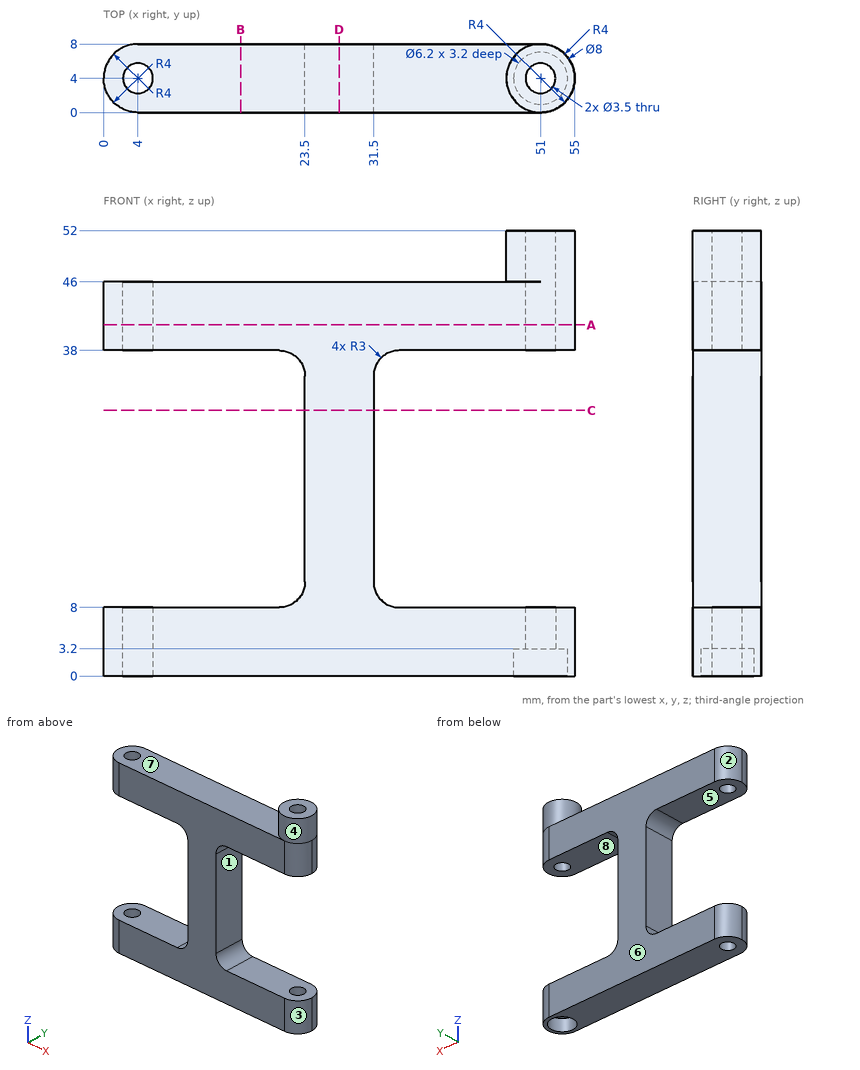
Geometry check sheet. Reference: drawing and pictorial views, mm from the part's lowest x, y, z. A direction names the side the tool comes from. Round coordinates to 2 decimals unless told otherwise and drop trailing zeros. Loops run counter-clockwise (first coordinate to the right, second up) from the corner with the lowest first, then second, coordinate; pieces in that order, holes last. Notation, with made-up numbers: (89.25, 13.25) - (93.25, 13.25) arc R27 ccw to (93.25, 48.25) - close; hole circle Ø4 at (19, 85). An arc over 180 degrees is marked (long way). Write item = value, one per line. Start each with the question number.
Q1. Section check C-C (z = 31). Record the boundary of the cut face in (x, y).
Q2. Section check A-A (z = 41). Count the separate pieces of the cut face and the enclosed holes in it, plus the area to 3 significant figures.
Q3. Section check B-B (x = 16). Record the boundary of the cut face in (y, z), plus the area to 3 significant figures.
Q4. Access from +Z, -Z, +X, -X, +Y, -Y to the whole of each face (thin tool, end or side, straight path). Record for the marked faces 1, 2, 3, 4 and 5.
Q5. Section check D-D (x = 27.5). Record the boundary of the cut face in (y, z), plus the area to 3 significant figures.
Q6. Depth check by flat-ended pin: P1, Ø4, axis at x = 4, y = 4, coming from the +Z side; P2, Ø4, axis at y = 6, z = 27.5, coming from the -X side. Enter the tip coordinate at first touch or a pass-through.
Q7. Thickness scan on L1, parallel to Z at x = 16.5, y = 3.75; L2, parallel to Y at x = 4, z = 5; L3, parallel to X at y = 3.75, z = 42. Record the ranges inside material, lowest first.
Q8. Release check for a two-part mould opening along Z. For the marked faces 6, 7 and 8 record: pulls with the +Z half, pulls with the -Z half, needs draft (parallel to the pull), parting line crosses it, or undercut.
Derived:
q1.outline = (23.5, 0) - (31.5, 0) - (31.5, 8) - (23.5, 8) - close
q2.separate_pieces = 1
q2.enclosed_holes = 2
q2.area = 407 mm^2
q3.outline = (0, 0) - (8, 0) - (8, 8) - (0, 8) - close; (0, 38) - (8, 38) - (8, 46) - (0, 46) - close
q3.area = 128 mm^2
q4.face_1 = +X, +Y, -Y
q4.face_2 = +Z, -Z, -X, +Y
q4.face_3 = +Z, -Z, +X, -Y
q4.face_4 = +Z
q4.face_5 = -X, +Y, -Y
q5.outline = (0, 0) - (8, 0) - (8, 46) - (0, 46) - close
q5.area = 368 mm^2
q6.P1 = 46
q6.P2 = 23.5
q7.L1 = 0 to 8, 38 to 46
q7.L2 = 0 to 2.25, 5.75 to 8
q7.L3 = 0.01 to 2.27, 5.73 to 49.27, 52.73 to 54.99
q8.face_6 = needs draft
q8.face_7 = pulls with the +Z half
q8.face_8 = undercut
